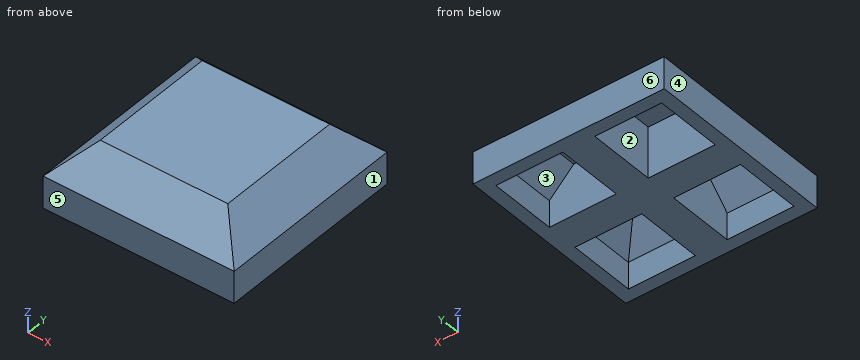
from build123d import *

# Parameters (mm, degrees)
SKETCH1_W           = 30
SKETCH1_H           = 30
BOSS_EXTRUDE1_DEPTH = 10
CHAMFER1_SIZE       = 5
SHELL1_T            = -2
BOSS_EXTRUDE2_REACH = 12


with BuildPart() as part:
    # Sketch1 → Boss-Extrude1 (new body)
    with BuildSketch(Plane.XY):
        Rectangle(SKETCH1_W, SKETCH1_H)
    extrude(amount=BOSS_EXTRUDE1_DEPTH)

    # Chamfer1
    chamfer1_edges = [part.edges().sort_by_distance(p)[0] for p in [
        (-15, 0, 10),
        (0, -15, 10),
        (15, 0, 10),
        (0, 15, 10),
    ]]
    chamfer(chamfer1_edges, length=CHAMFER1_SIZE)

    # Shell1
    shell1_openings = [part.faces().sort_by_distance(p)[0] for p in [
        (0, 0, 0),
    ]]
    offset(amount=SHELL1_T, openings=shell1_openings, kind=Kind.INTERSECTION)

    # Sketch2 → Boss-Extrude2 (add, up to next)
    with BuildSketch(Plane(origin=(0, 0, 0), x_dir=(-1, 0, 0), z_dir=(0, 0, -1)), mode=Mode.PRIVATE) as boss_extrude2_sk1:
        Polygon((13, 2.5), (2.5, 2.5), (2.5, 13), (-2.5, 13), (-2.5, 2.5), (-13, 2.5), (-13, -2.5), (-2.5, -2.5), (-2.5, -13), (2.5, -13), (2.5, -2.5), (13, -2.5), align=None)
    boss_extrude2_tool1 = extrude(boss_extrude2_sk1.sketch, amount=-BOSS_EXTRUDE2_REACH, mode=Mode.PRIVATE) - part.part
    add(boss_extrude2_tool1.solids().sort_by_distance((0, 0, 0))[0])


solid = part.part
Input: part model. Units: mm. Frame: model coordinates. Face numbers are marked on the shaded views. A direction names the side the tool comes from. Coordinates: 2 decimals unless noted, no trailing zeros. Order: outer loops, then holes, each group sorted by start corner. A loop starts at its lowest first (then second) coordinate and runs counter-clockwise, first axis right, second up.
1. Cut plane B-B, the plane y = -5.5. Return loops of the section in (x, z), plus the area to 3 significant figures.
Checked values:
outline: (-15, 0) - (-13, 0) - (-13, 4.17) - (-9.17, 8) - (-2.5, 8) - (-2.5, 0) - (2.5, 0) - (2.5, 8) - (9.17, 8) - (13, 4.17) - (13, 0) - (15, 0) - (15, 5) - (10, 10) - (-10, 10) - (-15, 5) - close
area: 122 mm2
2. Contact query for flat-ended pins moving along their axis: P1, Ø5.5, axis at x = 6.5, y = 5.5, coming from the -Z side; P2, Ø2, axis at x = -6, y = 6.5, coming from the -Z side; P3, Ø5.5, axis at x = -7.5, y = -5.5, coming from the -Z side. Output: stop coordinate, or through.
Checked values:
P1: stops at z = 7.92
P2: stops at z = 8
P3: stops at z = 6.92
3. Access query for the marked faces 1 and 2. Directions: +Z, -Z, +X, -X, +Y, -Y. A direction counts if a zero-diameter tool reaches every point of the face in a straight line with its end or side. Return the directions, or none.
Checked values:
face 1: +Z, -Z, +X, +Y, -Y
face 2: -Z
4. Ray query, line 1 along Y through (x, z) = (9, 2); line 2 along Y through (x, z) = (-8.5, 4.75). Return the intervals inside material, ascending.
Checked values:
line 1: y = -15 to -13, -2.5 to 2.5, 13 to 15
line 2: y = -15 to -12.42, -2.5 to 2.5, 12.42 to 15
5. Draft query along Y for the marked faces 3, 4, 5 and 6. Return one class per face: +Y half, -Y half, draft (parallel to the pull), parting line (faces both ways), or undercut.
Checked values:
face 3: undercut
face 4: draft
face 5: -Y half
face 6: +Y half
6. Cut plane D-D, the plane x = 0. Return loops of the section in (y, z), plus the area to 3 significant figures.
Checked values:
outline: (-15, 0) - (15, 0) - (15, 5) - (10, 10) - (-10, 10) - (-15, 5) - close
area: 275 mm2
7. Cut plane A-A, the plane z = 3.5. Return loops of the section in (x, y), plus the area to 3 significant figures.
Checked values:
outline: (-15, -15) - (15, -15) - (15, 15) - (-15, 15) - close; hole (-13, -13) - (-2.5, -13) - (-2.5, -2.5) - (-13, -2.5) - close; hole (-13, 2.5) - (-2.5, 2.5) - (-2.5, 13) - (-13, 13) - close; hole (2.5, -13) - (13, -13) - (13, -2.5) - (2.5, -2.5) - close; hole (2.5, 2.5) - (13, 2.5) - (13, 13) - (2.5, 13) - close
area: 459 mm2
